Autodesk Inventor part; units mm, degrees
ref_plane "YZ Plane" through (0, 0, 0) normal (1, 0, 0) x (0, 1, 0)
ref_plane "XZ Plane" through (0, 0, 0) normal (0, 1, 0) x (-1, 0, 0)
ref_plane "XY Plane" through (0, 0, 0) normal (0, 0, 1) x (1, 0, 0)
sketch "Skizze1" plane through (0, 0, 0) normal (0, 0, 1) x (1, 0, 0)
  line L0 (15, -15) -> (-15, -15)
  line L1 (-15, -15) -> (-15, 15)
  line L2 (-15, 15) -> (15, 15)
  line L3 (15, 15) -> (15, -15)
  line L4 (15, -15) -> (-15, 15) construction
  line L5 (-15, -15) -> (15, 15) construction
  line L6 (-7.5, -7.5) -> (7.5, -7.5) construction
  line L7 (7.5, -7.5) -> (7.5, 7.5) construction
  line L8 (7.5, 7.5) -> (-7.5, 7.5) construction
  line L9 (-7.5, 7.5) -> (-7.5, -7.5) construction
  line L10 (-7.5, -7.5) -> (7.5, 7.5) construction
  line L11 (7.5, -7.5) -> (-7.5, 7.5) construction
  circle A0 centre (-7.5, 7.5) radius 1.5
  circle A1 centre (7.5, 7.5) radius 1.5
  circle A2 centre (7.5, -7.5) radius 1.5
  circle A3 centre (-7.5, -7.5) radius 1.5
  circle A4 centre (0, 0) radius 1.3301
  dimension "d0" = 30
  dimension "d1" = 30
  dimension "d2" = 15
  dimension "d3" = 15
  dimension "d4" = 3
  dimension "d5" = 3
  dimension "d6" = 3
  dimension "d7" = 3
extrude "Extrusion1" add sketch "Skizze1" along normal blind 1
properties part number "00_Neopixel_4x4_Matrix"
The model under review builds one solid part; all positions refer to its coordinate system, in mm. Round coordinates to 2 decimals unless told otherwise and drop trailing zeros. Loops run counter-clockwise (first coordinate to the right, second up) from the corner with the lowest first, then second, coordinate; pieces in that order, holes last. Notation, with made-up numbers: M 54,32.25 L 76,32.25 A21 cw 76,60.25 Z; hole C 35.5,88 d7. An arc over 180 degrees is marked long. Answer as CSV lines item,"result". Start each with the question number.
Item 1: Consider section B-B (y = 0). Write out the cut boundary in (x, z), then the cut area to 3 significant figures.
Item 2: Mouldability with a two-part tool opening along Y and no side actions: class faces 1 (the face through (0.72, -1.12, 0.49)), 2 (the face through (-8.7, 8.4, 0.5)), 3 (the face through (-4, 0, 1)), 4 (the face through (0.2, -15, 0.5)) as released by +Y, released by -Y, zero draft, split by the parting line, or undercut.
Item 3: Wall thickness on line 1 (Y direction, x = -7.5, z = 0.4); line 2 (Y direction, x = -6.25, z = 0.3): over which ranges is each line inside the solid? List them lowest first. Write a range as [from, to].
Item 4: Consider section A-A (x = -7.5). Write out the cut boundary in (y, z), then the cut area to 3 significant figures.
Answer:
1,outline,"M -15,0 L -1.33,0 L -1.33,1 L -15,1 Z; M 1.33,0 L 15,0 L 15,1 L 1.33,1 Z"
1,area,"27.3 mm^2"
2,face 1,"undercut"
2,face 2,"undercut"
2,face 3,"zero draft"
2,face 4,"released by -Y"
3,line 1,"y = [-15, -9], [-6, 6], [9, 15]"
3,line 2,"y = [-15, -8.33], [-6.67, 6.67], [8.33, 15]"
4,outline,"M -15,0 L -9,0 L -9,1 L -15,1 Z; M -6,0 L 6,0 L 6,1 L -6,1 Z; M 9,0 L 15,0 L 15,1 L 9,1 Z"
4,area,"24.0 mm^2"
